Here's how the part is built. I have some questions about the finished solid (model axes, mm). A direction names the side the tool comes from. Coordinates: 2 decimals unless noted, no trailing zeros. Order: outer loops, then holes, each group sorted by start corner. A loop starts at its lowest first (then second) coordinate and runs counter-clockwise, first axis right, second up. Notation, with made-up numbers: (27, 22.5) - (66, 22.5) arc R24 cw to (66, 47.5) - close; hole circle Ø4 at (34.25, 34). An arc over 180 degrees is marked (long way). Answer as CSV lines item,"result". Start each with the question number.
Q1. For pin 1 Ø0.8 at (x, z) = (10, -3) entering from -Y; pin 2 Ø1 at (x, z) = (-10.5, -0.5) entering from +Y; pin 3 Ø6 at (x, z) = (-15.5, -3) entering from +Y, each with a flat end and sliding along its axis, tell me the tip position at first contact or that it passes through.
Q2. Suppose I cut it at C-C (y = 5). Please give me the cut outline in (x, z).
Q3. Thinking about a two-plate mould opening in Y: for faces 1 (the face through (7.955, 16.159, -4.056)), 2 (the face through (28, 1, -3)), 3 (the face through (23, -12, -3)), which applies, released by +Y, released by -Y, zero draft, split by the parting line, or undercut?
Q4. Suppose I cut it at B-B (x = 24.5). Please give me the cut outline in (y, z), then the cut area to 4 significant figures.
Q5. I need wall thicknesses on line 1 (X direction, y = 5, z = -2); line 2 (Y direction, x = 9, z = -2.25); line 3 (X direction, y = -7, z = -4). Which ranges of each line are inside material? Lowest first, please.
Q6. Suppose I cut it at D-D (x = 0). Please give me the cut outline in (y, z).
Q7. For faces 4 (the face through (23, 0, -3)), 5 (the face through (0, 12.65, -4)), 6 (the face through (20, 7, -3)), 7 (the face through (-0.4, 10.2, -8)), which set-ups out of +Z, -Z, +X, -X, +Y, -Y let a thin tool reach every point of the face, with its end or its side?
Q8. Suppose I cut it at A-A (y = -8). Please give me the cut outline in (x, z).
from build123d import *

# Parameters (mm, degrees)
EXTRUDE_3_DEPTH = 2
EXTRUDE_START   = -8
EXTRUDE_5_DEPTH = 8
FILLET_4_R      = 2


with BuildPart() as part:
    # Sketch 1 → Extrude 3 (new body)
    with BuildSketch(Plane.XY):
        Polygon((13, 14), (17.846153846, 14), (13, 18.5), align=None)
        Polygon((17.846153846, 14), (28, 14), (13, 18.5), align=None)
        Polygon((20, 12), (28, 12), (28, 14), (17.846153846, 14), align=None)
        Polygon((13, 12), (20, 12), (17.846153846, 14), (13, 14), align=None)
        Polygon((13, 14), (13, 18.5), (-3, 18.5), (-3, 14), (-2.136195996, 14), (-2.713546265, 15), (-1.356773133, 17.35), (1.356773133, 17.35), (2.713546265, 15), (7.286453735, 15), (8.643226867, 17.35), (11.356773133, 17.35), (12.713546265, 15), (12.136195996, 14), align=None)
        with BuildLine():
            Line((11.184271928, 14), (12.136195996, 14))
            Line((12.136195996, 14), (12.713546265, 15))
            Line((12.713546265, 15), (11.356773133, 17.35))
            Line((11.356773133, 17.35), (8.643226867, 17.35))
            Line((8.643226867, 17.35), (7.286453735, 15))
            Line((7.286453735, 15), (8.45, 15))
            ThreePointArc((8.45, 15), (10, 16.55), (11.55, 15))
            ThreePointArc((11.55, 15), (11.4556994, 14.467609865), (11.184271928, 14))
        make_face()
        with BuildLine():
            Line((11.356773133, 12.65), (12.136195996, 14))
            Line((12.136195996, 14), (11.184271928, 14))
            ThreePointArc((11.184271928, 14), (10, 13.45), (8.815728072, 14))
            Line((8.815728072, 14), (7.863804004, 14))
            Line((7.863804004, 14), (8.643226867, 12.65))
            Line((8.643226867, 12.65), (11.356773133, 12.65))
        make_face()
        with BuildLine():
            Line((7.863804004, 14), (8.815728072, 14))
            ThreePointArc((8.815728072, 14), (8.5443006, 14.467609865), (8.45, 15))
            Line((8.45, 15), (7.286453735, 15))
            Line((7.286453735, 15), (7.863804004, 14))
        make_face()
        Polygon((-3, 12), (13, 12), (13, 14), (12.136195996, 14), (11.356773133, 12.65), (8.643226867, 12.65), (7.863804004, 14), (2.136195996, 14), (1.356773133, 12.65), (-1.356773133, 12.65), (-2.136195996, 14), (-3, 14), align=None)
        Polygon((2.136195996, 14), (7.863804004, 14), (7.286453735, 15), (2.713546265, 15), align=None)
        with BuildLine():
            Line((-2.713546265, 15), (-2.136195996, 14))
            Line((-2.136195996, 14), (-1.184271928, 14))
            ThreePointArc((-1.184271928, 14), (-0.532390135, 16.4556994), (1.55, 15))
            Line((1.55, 15), (2.713546265, 15))
            Line((2.713546265, 15), (1.356773133, 17.35))
            Line((1.356773133, 17.35), (-1.356773133, 17.35))
            Line((-1.356773133, 17.35), (-2.713546265, 15))
        make_face()
        with BuildLine():
            Line((-1.184271928, 14), (-2.136195996, 14))
            Line((-2.136195996, 14), (-1.356773133, 12.65))
            Line((-1.356773133, 12.65), (1.356773133, 12.65))
            Line((1.356773133, 12.65), (2.136195996, 14))
            Line((2.136195996, 14), (1.184271928, 14))
            ThreePointArc((1.184271928, 14), (0, 13.45), (-1.184271928, 14))
        make_face()
        with BuildLine():
            ThreePointArc((1.55, 15), (1.4556994, 14.467609865), (1.184271928, 14))
            Line((1.184271928, 14), (2.136195996, 14))
            Line((2.136195996, 14), (2.713546265, 15))
            Line((2.713546265, 15), (1.55, 15))
        make_face()
        Polygon((-3, 18.5), (-28, 14), (-7.846153846, 14), align=None)
        Polygon((-3, 18.5), (-7.846153846, 14), (-3, 14), align=None)
        Polygon((-7.846153846, 14), (-10, 12), (-3, 12), (-3, 14), align=None)
        Polygon((-28, 14), (-28, 12), (-10, 12), (-7.846153846, 14), align=None)
        with BuildLine():
            Line((20, 10), (20, 5))
            Line((20, 5), (22.95, 5))
            ThreePointArc((22.95, 5), (24.5, 6.55), (26.05, 5))
            ThreePointArc((26.05, 5), (25.596015511, 3.903984489), (24.5, 3.45))
            Line((24.5, 3.45), (24.5, -3.45))
            ThreePointArc((24.5, -3.45), (25.596015511, -3.903984489), (26.05, -5))
            ThreePointArc((26.05, -5), (24.5, -6.55), (22.95, -5))
            Line((22.95, -5), (20, -5))
            Line((20, -5), (20, -10))
            Line((20, -10), (20, -12))
            Line((20, -12), (28, -12))
            Line((28, -12), (28, 12))
            Line((28, 12), (20, 12))
            Line((20, 12), (13, 12))
            Line((13, 12), (-3, 12))
            Line((-3, 12), (-10, 12))
            Line((-10, 12), (-28, 12))
            Line((-28, 12), (-28, -12))
            Line((-28, -12), (-20, -12))
            Line((-20, -12), (-20, -10))
            Line((-20, -10), (-20, -5))
            Line((-20, -5), (-22.95, -5))
            ThreePointArc((-22.95, -5), (-25.596015511, -6.096015511), (-24.5, -3.45))
            Line((-24.5, -3.45), (-24.5, 3.45))
            ThreePointArc((-24.5, 3.45), (-25.596015511, 6.096015511), (-22.95, 5))
            Line((-22.95, 5), (-20, 5))
            Line((-20, 5), (-20, 10))
            Line((-20, 10), (20, 10))
        make_face()
        with BuildLine():
            Line((-20, -5), (-20, 5))
            Line((-20, 5), (-22.95, 5))
            ThreePointArc((-22.95, 5), (-23.403984489, 3.903984489), (-24.5, 3.45))
            Line((-24.5, 3.45), (-24.5, -3.45))
            ThreePointArc((-24.5, -3.45), (-23.403984489, -3.903984489), (-22.95, -5))
            Line((-22.95, -5), (-20, -5))
        make_face()
        with BuildLine():
            Line((20, 5), (20, 3))
            ThreePointArc((20, 3), (22.121320344, 2.121320344), (23, 0))
            ThreePointArc((23, 0), (22.121320344, -2.121320344), (20, -3))
            Line((20, -3), (20, -5))
            Line((20, -5), (22.95, -5))
            ThreePointArc((22.95, -5), (23.403984489, -3.903984489), (24.5, -3.45))
            Line((24.5, -3.45), (24.5, 3.45))
            ThreePointArc((24.5, 3.45), (23.403984489, 3.903984489), (22.95, 5))
            Line((22.95, 5), (20, 5))
        make_face()
    extrude(amount=EXTRUDE_3_DEPTH)

    # Sketch 1_7 → Extrude 5 (add)
    with BuildSketch(Plane.XY.offset(EXTRUDE_START)):
        Polygon((13, 14), (13, 18.5), (-3, 18.5), (-3, 14), (-2.136195996, 14), (-2.713546265, 15), (-1.356773133, 17.35), (1.356773133, 17.35), (2.713546265, 15), (7.286453735, 15), (8.643226867, 17.35), (11.356773133, 17.35), (12.713546265, 15), (12.136195996, 14), align=None)
        Polygon((2.136195996, 14), (7.863804004, 14), (7.286453735, 15), (2.713546265, 15), align=None)
        Polygon((-3, 12), (13, 12), (13, 14), (12.136195996, 14), (11.356773133, 12.65), (8.643226867, 12.65), (7.863804004, 14), (2.136195996, 14), (1.356773133, 12.65), (-1.356773133, 12.65), (-2.136195996, 14), (-3, 14), align=None)
        Polygon((17.846153846, 14), (28, 14), (13, 18.5), align=None)
        Polygon((13, 14), (17.846153846, 14), (13, 18.5), align=None)
        Polygon((13, 12), (20, 12), (17.846153846, 14), (13, 14), align=None)
        Polygon((20, 12), (28, 12), (28, 14), (17.846153846, 14), align=None)
        Polygon((-3, 18.5), (-7.846153846, 14), (-3, 14), align=None)
        Polygon((-7.846153846, 14), (-10, 12), (-3, 12), (-3, 14), align=None)
        Polygon((-3, 18.5), (-28, 14), (-7.846153846, 14), align=None)
        Polygon((-28, 14), (-28, 12), (-10, 12), (-7.846153846, 14), align=None)
        with BuildLine():
            Line((20, 10), (20, 5))
            Line((20, 5), (22.95, 5))
            ThreePointArc((22.95, 5), (24.5, 6.55), (26.05, 5))
            ThreePointArc((26.05, 5), (25.596015511, 3.903984489), (24.5, 3.45))
            Line((24.5, 3.45), (24.5, -3.45))
            ThreePointArc((24.5, -3.45), (25.596015511, -3.903984489), (26.05, -5))
            ThreePointArc((26.05, -5), (24.5, -6.55), (22.95, -5))
            Line((22.95, -5), (20, -5))
            Line((20, -5), (20, -10))
            Line((20, -10), (20, -12))
            Line((20, -12), (28, -12))
            Line((28, -12), (28, 12))
            Line((28, 12), (20, 12))
            Line((20, 12), (13, 12))
            Line((13, 12), (-3, 12))
            Line((-3, 12), (-10, 12))
            Line((-10, 12), (-28, 12))
            Line((-28, 12), (-28, -12))
            Line((-28, -12), (-20, -12))
            Line((-20, -12), (-20, -10))
            Line((-20, -10), (-20, -5))
            Line((-20, -5), (-22.95, -5))
            ThreePointArc((-22.95, -5), (-25.596015511, -6.096015511), (-24.5, -3.45))
            Line((-24.5, -3.45), (-24.5, 3.45))
            ThreePointArc((-24.5, 3.45), (-25.596015511, 6.096015511), (-22.95, 5))
            Line((-22.95, 5), (-20, 5))
            Line((-20, 5), (-20, 10))
            Line((-20, 10), (20, 10))
        make_face()
        with BuildLine():
            Line((20, 5), (20, 3))
            ThreePointArc((20, 3), (22.121320344, 2.121320344), (23, 0))
            ThreePointArc((23, 0), (22.121320344, -2.121320344), (20, -3))
            Line((20, -3), (20, -5))
            Line((20, -5), (22.95, -5))
            ThreePointArc((22.95, -5), (23.403984489, -3.903984489), (24.5, -3.45))
            Line((24.5, -3.45), (24.5, 3.45))
            ThreePointArc((24.5, 3.45), (23.403984489, 3.903984489), (22.95, 5))
            Line((22.95, 5), (20, 5))
        make_face()
        with BuildLine():
            Line((-20, -5), (-20, 5))
            Line((-20, 5), (-22.95, 5))
            ThreePointArc((-22.95, 5), (-23.403984489, 3.903984489), (-24.5, 3.45))
            Line((-24.5, 3.45), (-24.5, -3.45))
            ThreePointArc((-24.5, -3.45), (-23.403984489, -3.903984489), (-22.95, -5))
            Line((-22.95, -5), (-20, -5))
        make_face()
    extrude(amount=EXTRUDE_5_DEPTH)

    # Fillet 4
    fillet_4_edges = [part.edges().sort_by_distance(p)[0] for p in [
        (13, 18.5, -3),
        (28, 14, -3),
        (28, -12, -3),
        (-28, -12, -3),
        (-28, 14, -3),
        (-3, 18.5, -3),
    ]]
    fillet(fillet_4_edges, radius=FILLET_4_R)


solid = part.part
Here are the results:
1,pin 1,"stops at y = 10"
1,pin 2,"stops at y = 17.24"
1,pin 3,"stops at y = 16.79"
2,outline,"(-28, -8) - (-26.05, -8) - (-26.05, 2) - (-28, 2) - close; (-22.95, -8) - (-20, -8) - (-20, 2) - (-22.95, 2) - close; (20, -8) - (22.95, -8) - (22.95, 2) - (20, 2) - close; (26.05, -8) - (28, -8) - (28, 2) - (26.05, 2) - close"
3,face 1,"undercut"
3,face 2,"zero draft"
3,face 3,"released by -Y"
4,outline,"(-12, -8) - (-6.55, -8) - (-6.55, 2) - (-12, 2) - close; (-3.45, -8) - (3.45, -8) - (3.45, 2) - (-3.45, 2) - close; (6.55, -8) - (15.05, -8) - (15.05, 2) - (6.55, 2) - close"
4,area,"208.5 mm²"
5,line 1,"x = -28 to -26.05, -22.95 to -20, 20 to 22.95, 26.05 to 28"
5,line 2,"y = 10 to 12.65, 17.35 to 18.5"
5,line 3,"x = -28 to -20, 20 to 28"
6,outline,"(10, -8) - (12.65, -8) - (12.65, 0) - (13.45, 0) - (13.45, 2) - (10, 2) - close; (16.55, 0) - (17.35, 0) - (17.35, -8) - (18.5, -8) - (18.5, 2) - (16.55, 2) - close"
7,face 4,"+Z, -Z"
7,face 5,"-Z"
7,face 6,"+Z, -Z, -Y"
7,face 7,"-Z, +X, -X, +Y, -Y"
8,outline,"(-28, -8) - (-20, -8) - (-20, 2) - (-28, 2) - close; (20, -8) - (28, -8) - (28, 2) - (20, 2) - close"
